Check sheet for the modelled part. Datum: model origin and axes. Units: mm. A direction names the side the tool comes from. Give positions to 0.01 mm unless a question says otherwise; leave off trailing zeros. Write each loop counter-clockwise with the first axis right and the second up, starting at its lowest first coordinate (ties: lowest second). Pieces come first, ordered by that corner, then holes. Notation, with made-up numbers: (-40, -1.5) -> (-34, -1.5) arc R25 ccw to (-34, 24.5) -> close; hole circle Ø2 at (77, 82.25). An arc over 180 degrees is marked (long way). Write each question's results on one line, items separated by ' | '. Start each with the question number.
```python
from build123d import *

# Parameters (mm, degrees)
F0_W     = 19.05
F0_H     = 19.05
F0_R     = 4.7625
F1_DEPTH = 12.7


with BuildPart() as f1:
    # F0 (on Front) → F1 (new body)
    with BuildSketch(Plane.XZ):
        with BuildLine():
            ThreePointArc((72.4011394938, -9.525), (72.8688679634, -4.7727043416), (73.025, 0))
            ThreePointArc((73.025, 0), (72.8688679634, 4.7727043416), (72.4011394938, 9.525))
            Line((72.4011394938, 9.525), (30.287569645, 9.525))
            ThreePointArc((30.287569645, 9.525), (31.3822627947, 4.8183069522), (31.75, 0))
            ThreePointArc((31.75, 0), (31.3822627947, -4.8183069522), (30.287569645, -9.525))
            Line((30.287569645, -9.525), (72.4011394938, -9.525))
        make_face()
        with BuildLine():
            Line((30.287569645, 9.525), (72.4011394938, 9.525))
            ThreePointArc((72.4011394938, 9.525), (51.6364726961, 51.6364726961), (9.525, 72.4011394938))
            Line((9.525, 72.4011394938), (9.525, 30.287569645))
            ThreePointArc((9.525, 30.287569645), (22.4506403027, 22.4506403027), (30.287569645, 9.525))
        make_face()
        with BuildLine():
            ThreePointArc((9.525, -72.4011394938), (51.6364726961, -51.6364726961), (72.4011394938, -9.525))
            Line((72.4011394938, -9.525), (30.287569645, -9.525))
            ThreePointArc((30.287569645, -9.525), (22.4506403027, -22.4506403027), (9.525, -30.287569645))
            Line((9.525, -30.287569645), (9.525, -72.4011394938))
        make_face()
        with BuildLine():
            Line((9.525, 30.287569645), (9.525, 72.4011394938))
            ThreePointArc((9.525, 72.4011394938), (0, 73.025), (-9.525, 72.4011394938))
            Line((-9.525, 72.4011394938), (-9.525, 30.287569645))
            ThreePointArc((-9.525, 30.287569645), (0, 31.75), (9.525, 30.287569645))
        make_face()
        with BuildLine():
            ThreePointArc((-9.525, -72.4011394938), (0, -73.025), (9.525, -72.4011394938))
            Line((9.525, -72.4011394938), (9.525, -30.287569645))
            ThreePointArc((9.525, -30.287569645), (0, -31.75), (-9.525, -30.287569645))
            Line((-9.525, -30.287569645), (-9.525, -72.4011394938))
        make_face()
        with BuildLine():
            Line((-9.525, 30.287569645), (-9.525, 72.4011394938))
            ThreePointArc((-9.525, 72.4011394938), (-51.6364726961, 51.6364726961), (-72.4011394938, 9.525))
            Line((-72.4011394938, 9.525), (-30.287569645, 9.525))
            ThreePointArc((-30.287569645, 9.525), (-22.4506403027, 22.4506403027), (-9.525, 30.287569645))
        make_face()
        with BuildLine():
            ThreePointArc((-72.4011394938, -9.525), (-51.6364726961, -51.6364726961), (-9.525, -72.4011394938))
            Line((-9.525, -72.4011394938), (-9.525, -30.287569645))
            ThreePointArc((-9.525, -30.287569645), (-22.4506403027, -22.4506403027), (-30.287569645, -9.525))
            Line((-30.287569645, -9.525), (-72.4011394938, -9.525))
        make_face()
        with BuildLine():
            Line((-30.287569645, 9.525), (-72.4011394938, 9.525))
            ThreePointArc((-72.4011394938, 9.525), (-73.025, 0), (-72.4011394938, -9.525))
            Line((-72.4011394938, -9.525), (-30.287569645, -9.525))
            ThreePointArc((-30.287569645, -9.525), (-31.75, 0), (-30.287569645, 9.525))
        make_face()
        with BuildLine():
            ThreePointArc((31.75, 0), (31.3822627947, 4.8183069522), (30.287569645, 9.525))
            Line((30.287569645, 9.525), (9.525, 9.525))
            Line((9.525, 9.525), (9.525, -9.525))
            Line((9.525, -9.525), (30.287569645, -9.525))
            ThreePointArc((30.287569645, -9.525), (31.3822627947, -4.8183069522), (31.75, 0))
        make_face()
        with BuildLine():
            Line((9.525, 9.525), (9.525, 30.287569645))
            ThreePointArc((9.525, 30.287569645), (0, 31.75), (-9.525, 30.287569645))
            Line((-9.525, 30.287569645), (-9.525, 9.525))
            Line((-9.525, 9.525), (9.525, 9.525))
        make_face()
        with BuildLine():
            Line((-9.525, -9.525), (-9.525, 9.525))
            Line((-9.525, 9.525), (-30.287569645, 9.525))
            ThreePointArc((-30.287569645, 9.525), (-31.75, 0), (-30.287569645, -9.525))
            Line((-30.287569645, -9.525), (-9.525, -9.525))
        make_face()
        Rectangle(F0_W, F0_H)
        Circle(F0_R, mode=Mode.SUBTRACT)
        with BuildLine():
            ThreePointArc((-9.525, -30.287569645), (0, -31.75), (9.525, -30.287569645))
            Line((9.525, -30.287569645), (9.525, -9.525))
            Line((9.525, -9.525), (-9.525, -9.525))
            Line((-9.525, -9.525), (-9.525, -30.287569645))
        make_face()
    extrude(amount=F1_DEPTH)


solid = f1.part
```
Item 1: Mould release check, pull along X, two halves, no side actions. Record for faces 1 (the cylindrical face through (22.3, -6.3, 22.6)), 2 (the flat face through (15, -12.7, 1)): pulls with the +X half, pulls with the -X half, needs draft (parallel to the pull), parting line crosses it, or undercut.
Item 2: Thickness scan on probe 1 along Z at (x, y) = (0, -5.25) (1 decimal); probe 2 along Z at (x, y) = (23.5, -10.75) (3 decimals); probe 3 along X at (y, z) = (-5, -0.5). Record the ranges inside material, lowest first. Write a range as from..to.
Item 3: Depth check by flat-ended pin: pin 1 Ø4 at (y, z) = (-10.5, -48.5) entering from +X; pin 2 Ø4 at (y, z) = (-3.5, 23) entering from -X; pin 3 Ø6 at (x, y) = (-23.5, -10) entering from -Z. Enter the tip coordinate at first touch or a pass-through.
Item 4: Set-up check for faces 3 (the flat face through (15, 0, 1)), 4 (the flat face through (20, -6, 9.525)): record each of +Z, -Z, +X, -X, +Y, -Y from which the full face is reachable in a straight line by a thin tool's end or side.
Item 5: Section check B-B on y = -2. Count the separate pieces of the cut face and the enclosed holes in it, then the cut area to 3 significant figures.
Item 6: Section check A-A on x = 0. Record the boundary of the cut face in (y, z) (1 decimal), then the cut area to 3 significant figures.
Item 7: Section check D-D on z = -52.5. Record the boundary of the cut face in (x, y).
Item 8: Section check C-C on x = 21. Record the boundary of the cut face in (y, z) (3 decimals).
Check sheet entries:
1) face 1: undercut | face 2: needs draft
2) probe 1: z = -73..-4.8, 4.8..73 | probe 2: z = -69.14..-21.35, -9.525..9.525, 21.35..69.14 | probe 3: x = -73.02..-4.74, 4.74..73.02
3) pin 1: stops at x = 56.31 | pin 2: stops at x = -69.94 | pin 3: stops at z = -70.09
4) face 3: +Z, -Z, +X, -X, +Y | face 4: +Y, -Y
5) separate pieces: 1 | enclosed holes: 5 | area: 15,500 mm^2
6) outline: (-12.7, -73) -> (0, -73) -> (0, -4.8) -> (-12.7, -4.8) -> close; (-12.7, 4.8) -> (0, 4.8) -> (0, 73) -> (-12.7, 73) -> close | area: 1,730 mm^2
7) outline: (-50.76, -12.7) -> (50.76, -12.7) -> (50.76, 0) -> (-50.76, 0) -> close
8) outline: (-12.7, -69.94) -> (0, -69.94) -> (0, -23.813) -> (-12.7, -23.813) -> close; (-12.7, -9.525) -> (0, -9.525) -> (0, 9.525) -> (-12.7, 9.525) -> close; (-12.7, 23.813) -> (0, 23.813) -> (0, 69.94) -> (-12.7, 69.94) -> close
